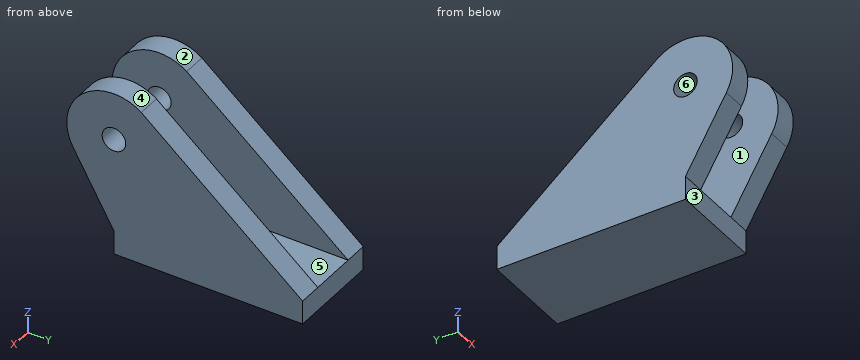
from build123d import *

# Parameters (mm, degrees)
SKETCH1_W           = 25.4
SKETCH1_H           = 50.8
BOSS_EXTRUDE1_DEPTH = 6.35
SKETCH2_R           = 3.175
BOSS_EXTRUDE2_DEPTH = 6.35
SKETCH3_R           = 3.175
BOSS_EXTRUDE3_DEPTH = 6.35


with BuildPart() as part:
    # Sketch1 → Boss-Extrude1 (new body)
    with BuildSketch(Plane.XY):
        with Locations((12.7, 25.4)):
            Rectangle(SKETCH1_W, SKETCH1_H)
    extrude(amount=BOSS_EXTRUDE1_DEPTH)

    # Sketch2 → Boss-Extrude2 (add)
    with BuildSketch(Plane(origin=(25.4, 0, 0), x_dir=(0, 0, -1), z_dir=(1, 0, 0))):
        with BuildLine():
            Line((-6.35, 0), (-25.4, -10.998522628))
            ThreePointArc((-25.4, -10.998522628), (-41.146035344, -8.544268244), (-42.097436971, 7.363460336))
            Line((-42.097436971, 7.363460336), (-6.35, 50.8))
            Line((-6.35, 50.8), (-6.35, 0))
        make_face()
        with Locations((-31.75, 0)):
            Circle(SKETCH2_R, mode=Mode.SUBTRACT)
    extrude(amount=-BOSS_EXTRUDE2_DEPTH)

    # Sketch3 → Boss-Extrude3 (add)
    with BuildSketch(Plane.ZY):
        with BuildLine():
            Line((6.35, 0), (25.4, -10.998522628))
            ThreePointArc((25.4, -10.998522628), (41.146035344, -8.544268244), (42.097436971, 7.363460336))
            Line((42.097436971, 7.363460336), (6.35, 50.8))
            Line((6.35, 50.8), (6.35, 0))
        make_face()
        with Locations((31.75, 0)):
            Circle(SKETCH3_R, mode=Mode.SUBTRACT)
    extrude(amount=-BOSS_EXTRUDE3_DEPTH)


solid = part.part
The model under review builds one solid part; all positions refer to its coordinate system, in mm. Face numbers are marked on the shaded views. A direction names the side the tool comes from. Round coordinates to 2 decimals unless told otherwise and drop trailing zeros. Order: outer loops, then holes, each group sorted by start corner. A loop starts at its lowest first (then second) coordinate and runs counter-clockwise, first axis right, second up. Notation, with made-up numbers: (-2, 65.25) - (51, 65.25) arc R14 cw to (51, 89.25) - close; hole circle Ø7 at (-24, 84.25). An arc over 180 degrees is marked (long way). Use one line per item in the form item = value.
Q1. Mouldability with a two-part tool opening along Z and no side actions: class the marked faces 4, 5 and 6 as pulls with the +Z half, pulls with the -Z half, needs draft (parallel to the pull), parting line crosses it, or undercut.
Response values:
face_4 = parting line crosses it
face_5 = pulls with the +Z half
face_6 = undercut
Q2. Add section B-B on z = 31.75. Give the boundary of the cut face in (x, y) (3 decimals), then the cut area to 3 significant figures.
Response values:
outline = (0, -12.7) - (6.35, -12.7) - (6.35, -3.175) - (0, -3.175) - close; (0, 3.175) - (6.35, 3.175) - (6.35, 19.937) - (0, 19.937) - close; (19.05, -12.7) - (25.4, -12.7) - (25.4, -3.175) - (19.05, -3.175) - close; (19.05, 3.175) - (25.4, 3.175) - (25.4, 19.937) - (19.05, 19.937) - close
area = 334 mm^2
Q3. Clearance check with flat-ended pins moving along their axes: P1, Ø12, axis at x = 14, z = 6, coming from the -Y side; P2, Ø1.5, axis at x = 8, z = 21.5, coming from the +Y side; P3, Ø1.9, axis at x = 18.5, z = 2.5, coming from the -Y side; P4, Ø3, axis at x = 4, y = 25, coming from the +Z side. State where each tip first meets the part, or that it passes through.
Response values:
P1 = -1.67
P2 = through
P3 = 0
P4 = 28.82
Q4. Tool access review of the marked faces 1, 2 and 3: name each direction out of +Z, -Z, +X, -X, +Y, -Y from which nothing blocks a thin tool from reaching the whole face with its end or side.
Response values:
face_1 = +Z, +Y, -Y
face_2 = +X, -X
face_3 = -Z, +X, -X, -Y
Q5. Add section C-C on z = 24. Give the boundary of the cut face in (x, y).
Response values:
outline = (0, -10.19) - (6.35, -10.19) - (6.35, 29.35) - (0, 29.35) - close; (19.05, -10.19) - (25.4, -10.19) - (25.4, 29.35) - (19.05, 29.35) - close
Q6. Add section A-A on x = 21.5. Give the boundary of the cut face in (y, z) (3 decimals).
Response values:
outline = (-10.999, 25.4) - (0, 6.35) - (0, 0) - (50.8, 0) - (50.8, 6.35) - (7.363, 42.097) arc R12.7 ccw to start; hole circle Ø6.35 at (0, 31.75)
Q7. To check wall thickness, follow line 1 (X direction, y = 7.5, z = 31); line 2 (Y direction, x = 21, z = 31.75) (3 decimals); line 3 (Y direction, x = 18.5, z = 5.5). State the ranges of each line that lie inside material, in increasing order.
Response values:
line_1 = 0 to 6.35, 19.05 to 25.4
line_2 = -12.7 to -3.175, 3.175 to 19.937
line_3 = 0 to 50.8
Q8. Add section D-D on y = 22.5. Give the boundary of the cut face in (x, z), then the cut area to 3 significant figures.
Response values:
outline = (0, 0) - (25.4, 0) - (25.4, 29.64) - (19.05, 29.64) - (19.05, 6.35) - (6.35, 6.35) - (6.35, 29.64) - (0, 29.64) - close
area = 457 mm^2
